The listing builds one solid part. Answer for the finished solid, in the listing's coordinates (mm). A direction names the side the tool comes from. Give positions to 0.01 mm unless a question says otherwise; leave off trailing zeros. Order: outer loops, then holes, each group sorted by start corner. A loop starts at its lowest first (then second) coordinate and runs counter-clockwise, first axis right, second up. Notation, with made-up numbers: (-30.75, 43) - (5.25, 43) arc R16 ccw to (5.25, 71) - close; hole circle Ø6 at (56.25, 33). An arc over 180 degrees is marked (long way). Use a Markdown table: item, result. Add a question column.
1) Find section B-B, the plane x = 12. Determine the outline of the cut face in (y, z), plus the area to 3 significant figures.
2) Find section C-C, the plane z = 14. Determine the outline of the cut face in (x, y).
3) For faces 4 (the face through (28.2, -1, -31)), 5 (the face through (91, -2, -5)), 6 (the face through (98.1, -1, 28)), determine the directions among +Z, -Z, +X, -X, +Y, -Y from which every point of the face is accessible in a straight line to the end or side of a thin tool.
4) Straight lines are drawn through the part: line 1 (X direction, y = -2.6, z = 19.5); line 2 (X direction, y = -1, z = -3); line 3 (X direction, y = -1.9, z = 22). For each, find the intervals that lie inside material, in ascending order.
5) The mould has two halves that part along X. Classify faces 1 (the face through (69.1, -1, -32)), 2 (the face through (98.1, -1, -28)), 3 (the face through (51, -3, 22)): released by +X, released by -X, zero draft, split by the parting line, or undercut.
6) Find section A-A, the plane z = -1.5. Determine the outline of the cut face in (x, y), plus the area to 3 significant figures.
7) Flat-ended cylindrical pins translate along their axes: pin 1 (0.9 mm diameter, centred on x = 90.5, y = -1, fed in from +Z); pin 2 (1 mm diameter, centred on x = 39.5, y = -0.5, fed in from -Z); pin 3 (0.9 mm diameter, centred on y = -1, z = -27, fed in from +X). Find the tip coordinate at first contact, or state that the pin passes through.
8) Find section D-D, the plane y = -0.65. State how many separate pieces and enclosed holes the cut face has, plus the area to 3 significant figures.
from build123d import *

# Parameters (mm, degrees)
BOSS_EXTRUDE1_DEPTH = 3
SKETCH2_W           = 41.5
SKETCH2_H           = 43.04695539
CUT_EXTRUDE1_DEPTH  = 3


with BuildPart() as part:
    # Sketch1 → Boss-Extrude1 (new body)
    with BuildSketch(Plane(origin=(0, 0, 0), x_dir=(1, 0, 0), z_dir=(0, 1, 0))):
        Polygon((0, -28.5), (0, 28.5), (13.2, 28.836391437), (13.2, 31.837365446), (28.2, 32.219628443), (28.2, 29.218654434), (69.1, 30.260958206), (69.1, 33.261932214), (83.1, 33.618711012), (83.1, 30.617737003), (98.1, 31), (98.1, 25), (101.1, 25), (101.1, -25), (98.1, -25), (98.1, -31), (83.1, -30.617737003), (83.1, -33.618711012), (69.1, -33.261932214), (69.1, -30.260958206), (28.2, -29.218654434), (28.2, -32.219628443), (13.2, -31.837365446), (13.2, -28.836391437), align=None)
    extrude(amount=-BOSS_EXTRUDE1_DEPTH)

    # Sketch2 → Cut-Extrude1 (cut)
    with BuildSketch(Plane.XZ.offset(3)):
        Polygon((60.95, 22.300745789), (60.95, -22.300745789), (81.45, -22.823171885), (81.45, 22.823171885), align=None)
        Polygon((93.95, 0), (93.95, 5), (88.95, 5), (88.95, -5), (93.95, -5), align=None)
        with Locations((30.45, -0.528797146)):
            Rectangle(SKETCH2_W, SKETCH2_H)
    extrude(amount=-CUT_EXTRUDE1_DEPTH, mode=Mode.SUBTRACT)


solid = part.part
The answers:
| question | item | result |
|---|---|---|
| 1 | outline | (-3, -28.81) - (0, -28.81) - (0, -22.05) - (-3, -22.05) - close; (-3, 20.99) - (0, 20.99) - (0, 28.81) - (-3, 28.81) - close |
| 1 | area | 43.7 mm2 |
| 2 | outline | (0, -3) - (9.7, -3) - (9.7, 0) - (0, 0) - close; (51.2, -3) - (60.95, -3) - (60.95, 0) - (51.2, 0) - close; (81.45, -3) - (101.1, -3) - (101.1, 0) - (81.45, 0) - close |
| 3 | face 4 | -Z, +Y, -Y |
| 3 | face 5 | +Y, -Y |
| 3 | face 6 | +Z, +X, +Y, -Y |
| 4 | line 1 | 0 to 9.7, 51.2 to 60.95, 81.45 to 101.1 |
| 4 | line 2 | 0 to 9.7, 51.2 to 60.95, 81.45 to 88.95, 93.95 to 101.1 |
| 4 | line 3 | 0 to 60.95, 81.45 to 101.1 |
| 5 | face 1 | undercut |
| 5 | face 2 | released by +X |
| 5 | face 3 | zero draft |
| 6 | outline | (0, -3) - (9.7, -3) - (9.7, 0) - (0, 0) - close; (51.2, -3) - (60.95, -3) - (60.95, 0) - (51.2, 0) - close; (81.45, -3) - (88.95, -3) - (88.95, 0) - (81.45, 0) - close; (93.95, -3) - (101.1, -3) - (101.1, 0) - (93.95, 0) - close |
| 6 | area | 102 mm2 |
| 7 | pin 1 | z = 30.82 |
| 7 | pin 2 | z = -29.52 |
| 7 | pin 3 | x = 98.1 |
| 8 | separate pieces | 1 |
| 8 | enclosed holes | 3 |
| 8 | area | 3,400 mm2 |
